Geometry check sheet. Reference: the model listing, model coordinates, mm. A direction names the side the tool comes from. Round coordinates to 2 decimals unless told otherwise and drop trailing zeros. Loops run counter-clockwise (first coordinate to the right, second up) from the corner with the lowest first, then second, coordinate; pieces in that order, holes last. Notation, with made-up numbers: M 65.5,49.5 L 72.5,49.5 A25 cw 72.5,78.5 Z; hole C -15.75,-8.5 d7. An arc over 180 degrees is marked long. Use one line per item in the form item = value. Start each with the question number.
1. Go/stop test with flat-tipped pins: pin 1 (1 mm diameter, centred on y = 2, z = 4.5, fed in from +X); pin 2 (4.5 mm diameter, centred on x = -6.5, z = 5.5, fed in from +Y). Record where each tip stops, or that it passes through.
2. Cross-section at C-C (z = 3.25). Record the boundary of the cut face in (x, y).
3. Cross-section at B-B (x = -8.25). Record the boundary of the cut face in (y, z).
4. Material ranges on line 1 (Z direction, x = -0.5, y = 5.5); line 2 (Y direction, x = -5.25, z = 9.5); line 3 (X direction, y = 4.75, z = 2.25), recorded low to high.
5. Set-up check for faces 1 (the flat face through (-5, 1, 5)), 2 (the flat face through (-5, 0, 5)): record each of +Z, -Z, +X, -X, +Y, -Y from which the full face is reachable in a straight line by a thin tool's end or side.
6. Cross-section at A-A (y = 3.25). Record the boundary of the cut face in (x, z).
7. Draft check along Z on faces 3 (the flat face through (-10, 4, 5)), 4 (the flat face through (-5, 4, 0)), 5 (the flat face through (-5, 5, 10)). Enter one of: pulls with the +Z half, pulls with the -Z half, needs draft (parallel to the pull), parting line crosses it, or undercut.
```python
from build123d import *

# Parameters (mm, degrees)
BOX102_W     = 9
BOX102_H     = 8
BOX102_DEPTH = 1
BOX005_W     = 8
BOX005_H     = 1
BOX005_DEPTH = 11
BOX006_W     = 9
BOX006_H     = 1
BOX006_DEPTH = 11
BOX100_W     = 9
BOX100_H     = 7
BOX100_DEPTH = 1


with BuildPart() as box102:
    # Box102 → Box102 (new body)
    with BuildSketch(Plane(origin=(-9, 0, 0), x_dir=(1, 0, 0), z_dir=(0, 0, 1))):
        with Locations((4.5, 4)):
            Rectangle(BOX102_W, BOX102_H)
    extrude(amount=BOX102_DEPTH)


with BuildPart() as box005:
    # Box005 → Box005 (new body)
    with BuildSketch(Plane(origin=(-9, 0, 0), x_dir=(0, 1, 0), z_dir=(0, 0, 1))):
        with Locations((4, 0.5)):
            Rectangle(BOX005_W, BOX005_H)
    extrude(amount=BOX005_DEPTH)


with BuildPart() as box006:
    # Box006 → Box006 (new body)
    with BuildSketch(Plane(origin=(-9, 0, 0), x_dir=(1, 0, 0), z_dir=(0, 0, 1))):
        with Locations((4.5, 0.5)):
            Rectangle(BOX006_W, BOX006_H)
    extrude(amount=BOX006_DEPTH)


with BuildPart() as fusion043:
    # Box100 → Box100 (new body)
    with BuildSketch(Plane(origin=(-9, 1, 10), x_dir=(1, 0, 0), z_dir=(0, 0, 1))):
        with Locations((4.5, 3.5)):
            Rectangle(BOX100_W, BOX100_H)
    extrude(amount=BOX100_DEPTH)

    # Fusion041: union Box006
    add(box006.part)

    # Fusion042: union Box005
    add(box005.part)

    # Fusion043: union Box102
    add(box102.part)


solid = fusion043.part
```
Reported:
q1.pin_1 = -9
q1.pin_2 = 1
q2.outline = M -10,0 L 0,0 L 0,1 L -9,1 L -9,8 L -10,8 Z
q3.outline = M 0,0 L 8,0 L 8,1 L 1,1 L 1,10 L 8,10 L 8,11 L 0,11 Z
q4.line_1 = 0 to 1, 10 to 11
q4.line_2 = 0 to 1
q4.line_3 = -10 to -9
q5.face_1 = +X, +Y
q5.face_2 = +Z, -Z, +X, -X, -Y
q6.outline = M -10,0 L 0,0 L 0,1 L -9,1 L -9,10 L 0,10 L 0,11 L -10,11 Z
q7.face_3 = needs draft
q7.face_4 = pulls with the -Z half
q7.face_5 = undercut
